```python
from build123d import *

# Parameters (mm, degrees)
SKETCH1_W               = 100
SKETCH1_H               = 240
SKETCH1_R               = 8
SKETCH1_R_2             = 10
BOSS_EXTRUDE1_DEPTH     = 25
SKETCH2_OUTSIDE_W       = 154.952
SKETCH2_OUTSIDE_H       = 294.952
SKETCH2_OUTSIDE_R       = 10
SKETCH2_OUTSIDE_R_2     = 8
CUT_EXTRUDE1_DEPTH      = 10
CUT_EXTRUDE2_START      = -50
SKETCH3_OUTSIDE_W       = 154.952
SKETCH3_OUTSIDE_H       = 294.952
CUT_EXTRUDE2_DEPTH      = 50
CUT_EXTRUDE7_REACH      = 242
SKETCH8_R               = 8
BOSS_EXTRUDE2_DEPTH     = 30
CUT_EXTRUDE8_REACH      = 242
CUT_EXTRUDE8_END_RADIUS = 115
CUT_EXTRUDE9_START      = -25.8
SKETCH10_R              = 5
CUT_EXTRUDE9_DEPTH      = 25.8
LPATTERN1_COUNT         = 4
LPATTERN1_PITCH         = 55
MIRROR1_START           = -25.8
MIRROR1_COPY_1_SKETCH_R = 5
MIRROR1_COPY_1_DEPTH    = 25.8
MIRROR1_COPY_2_SKETCH_R = 5
MIRROR1_COPY_2_DEPTH    = 25.8
MIRROR1_COPY_3_SKETCH_R = 5
MIRROR1_COPY_3_DEPTH    = 25.8
FILLET1_R               = 5


with BuildPart() as part:
    # Sketch1 → Boss-Extrude1 (new body, symmetric)
    with BuildSketch(Plane.XY):
        Rectangle(SKETCH1_W, SKETCH1_H)
        with Locations((0, 3)):
            Circle(SKETCH1_R, mode=Mode.SUBTRACT)
        with Locations((0, -85)):
            Circle(SKETCH1_R_2, mode=Mode.SUBTRACT)
    extrude(amount=BOSS_EXTRUDE1_DEPTH, both=True)

    # Sketch2 outside → Cut-Extrude1 (cut)
    with BuildSketch(Plane.XY.offset(25)):
        Rectangle(SKETCH2_OUTSIDE_W, SKETCH2_OUTSIDE_H)
        with BuildLine():
            Line((50, -120), (50, 18.561575886))
            ThreePointArc((50, 18.561575886), (0, 30), (-50, 18.561575886))
            Line((-50, 18.561575886), (-50, -120))
            Line((-50, -120), (50, -120))
        make_face(mode=Mode.SUBTRACT)
        with Locations((0, -85)):
            Circle(SKETCH2_OUTSIDE_R)
        with Locations((0, 3)):
            Circle(SKETCH2_OUTSIDE_R_2)
    extrude(amount=-CUT_EXTRUDE1_DEPTH, mode=Mode.SUBTRACT)

    # Sketch3 outside → Cut-Extrude2 (cut)
    with BuildSketch(Plane.XY.offset(25).offset(CUT_EXTRUDE2_START)):
        Rectangle(SKETCH3_OUTSIDE_W, SKETCH3_OUTSIDE_H)
        with BuildLine():
            Line((50, 120), (-50, 120))
            Line((-50, 120), (-50, -109.378823628))
            ThreePointArc((-50, -109.378823628), (0, -120), (50, -109.378823628))
            Line((50, -109.378823628), (50, 120))
        make_face(mode=Mode.SUBTRACT)
    extrude(amount=CUT_EXTRUDE2_DEPTH, mode=Mode.SUBTRACT)

    # Sketch7 → Cut-Extrude7 (cut, up to next)
    with BuildSketch(Plane(origin=(0, 120, 0), x_dir=(1, 0, 0), z_dir=(0, 1, 0)), mode=Mode.PRIVATE) as cut_extrude7_sk1:
        Polygon((-35, 0), (35, 0), (20, 25), (-20, 25), align=None)
    cut_extrude7_tool1 = extrude(cut_extrude7_sk1.sketch, amount=-CUT_EXTRUDE7_REACH, mode=Mode.PRIVATE) & part.part
    add(cut_extrude7_tool1.solids().sort_by_distance((0, 120, -11.363636))[0], mode=Mode.SUBTRACT)

    # Sketch8 → Boss-Extrude2 (add)
    with BuildSketch(Plane(origin=(0, 120, 0), x_dir=(1, 0, 0), z_dir=(0, 1, 0))):
        with BuildLine():
            Line((13, 15), (13, 0))
            Line((13, 0), (-13, 0))
            Line((-13, 0), (-13, 15))
            ThreePointArc((-13, 15), (0, 28), (13, 15))
        make_face()
        with Locations(Location((0, 15, 0), (0, 0, 270))):  # turned: the seam where the file's is
            Circle(SKETCH8_R, mode=Mode.SUBTRACT)
    extrude(amount=-BOSS_EXTRUDE2_DEPTH)

    # Cut-Extrude8: up to this cylinder (the profile starts outside it)
    cut_extrude8_end = Plane(origin=(0, -85, 18.800927), z_dir=(0, 0, 1)) * Cylinder(CUT_EXTRUDE8_END_RADIUS, 715, mode=Mode.PRIVATE)
    # Sketch9 → Cut-Extrude8 (cut, up to the surface)
    with BuildSketch(Plane(origin=(0, 120, 0), x_dir=(1, 0, 0), z_dir=(0, 1, 0)), mode=Mode.PRIVATE) as cut_extrude8_sk1:
        with BuildLine():
            Line((50, -8.64916731), (50, -25))
            Line((50, -25), (-50, -25))
            Line((-50, -25), (-50, -8.64916731))
            ThreePointArc((-50, -8.64916731), (0, -15), (50, -8.64916731))
        make_face()
    cut_extrude8_tool1 = extrude(cut_extrude8_sk1.sketch, amount=-CUT_EXTRUDE8_REACH, mode=Mode.PRIVATE) - cut_extrude8_end
    add(cut_extrude8_tool1.solids().sort_by_distance((0, 120, 18.800927))[0], mode=Mode.SUBTRACT)

    # Sketch10 → Cut-Extrude9 (cut)
    with BuildSketch(Plane(origin=(50, 0, 0), x_dir=(0, 0, -1), z_dir=(1, 0, 0)).offset(CUT_EXTRUDE9_START)):
        with Locations((13, -90)):
            Circle(SKETCH10_R)
    cut_extrude9 = extrude(amount=CUT_EXTRUDE9_DEPTH, mode=Mode.SUBTRACT)

    # LPattern1: Cut-Extrude9 ×4
    with Locations(*[(0, i * LPATTERN1_PITCH, 0) for i in range(1, LPATTERN1_COUNT)]):
        add(cut_extrude9, mode=Mode.SUBTRACT)

    # Mirror1: Cut-Extrude9 across plane
    add(cut_extrude9.mirror(Plane(origin=(0, 0, 0), x_dir=(0, 0, 1), z_dir=(1, 0, 0))), mode=Mode.SUBTRACT)

    # Mirror1 copy 1 sketch → Mirror1 copy 1 (cut)
    with BuildSketch(Plane(origin=(-50, 55, 0), x_dir=(0, 0, -1), z_dir=(-1, 0, 0)).offset(MIRROR1_START)):
        with Locations((13, 90)):
            Circle(MIRROR1_COPY_1_SKETCH_R)
    extrude(amount=MIRROR1_COPY_1_DEPTH, mode=Mode.SUBTRACT)

    # Mirror1 copy 2 sketch → Mirror1 copy 2 (cut)
    with BuildSketch(Plane(origin=(-50, 110, 0), x_dir=(0, 0, -1), z_dir=(-1, 0, 0)).offset(MIRROR1_START)):
        with Locations((13, 90)):
            Circle(MIRROR1_COPY_2_SKETCH_R)
    extrude(amount=MIRROR1_COPY_2_DEPTH, mode=Mode.SUBTRACT)

    # Mirror1 copy 3 sketch → Mirror1 copy 3 (cut)
    with BuildSketch(Plane(origin=(-50, 165, 0), x_dir=(0, 0, -1), z_dir=(-1, 0, 0)).offset(MIRROR1_START)):
        with Locations((13, 90)):
            Circle(MIRROR1_COPY_3_SKETCH_R)
    extrude(amount=MIRROR1_COPY_3_DEPTH, mode=Mode.SUBTRACT)

    # Fillet1
    fillet1_edges = [part.edges().sort_by_distance(p)[0] for p in [
        (-1e-09, 30, 15),
    ]]
    fillet(fillet1_edges, radius=FILLET1_R)


solid = part.part
```
Work out the finished part from the listing and answer in its coordinate system (mm). A direction names the side the tool comes from. Give positions to 0.01 mm unless a question says otherwise; leave off trailing zeros. Loops run counter-clockwise (first coordinate to the right, second up) from the corner with the lowest first, then second, coordinate; pieces in that order, holes last. Notation, with made-up numbers: (30, 61) -> (35, 61) arc R10 cw to (35, 66) -> close; hole circle Ø4 at (41.5, 58.25). An arc over 180 degrees is marked (long way). Put each result on its own line as item: value. Start each with the question number.
Item 1: The part is cut by section A-A (y = 75). Give the vertices of the cut face in (x, z), then the cut area to 3 significant figures.
Item 2: The mould has two halves that part along Z. Classify faces 4 (the face through (-35, 2, -25)), 5 (the face through (39.786, -36.915, -17.619)), 6 (the face through (50, 4, -5)): released by +Z, released by -Z, zero draft, split by the parting line, or undercut.
Item 3: Each of these flat-tipped pins is pushed along its axis until it touches: P1, Ø1, axis at x = 34.5, z = -17, coming from the -Y side; P2, Ø21, axis at x = 14, y = 36.5, coming from the -Z side; P3, Ø8, axis at x = 5.5, y = 70, coming from the +Z side. Where does it stop, or does it pass through?
Item 4: The part is cut by section C-C (y = 105). Give the vertices of the cut face in (x, z).
Item 5: Which of the six approach directions +Z, -Z, +X, -X, +Y, -Y give full straight-line access (tool end or side, diameter ignored) to faces 1 (the face through (6, 90, -8)), 2 (the face through (13, 105, -8)), 3 (the face through (-8.3, 1.7, 0))?
Item 6: The part is cut by section D-D (y = -102). Give the vertices of the cut face in (x, z), then the cut area to 4 significant figures.
Item 7: The part is cut by section B-B (z = 22.5). Give the vertices of the cut face in (x, y), then the cut area to 3 significant figures.
Item 8: Find the intervals of material crossed by L1, parallel to Z at x = -36.75, y = -35; L2, parallel to X at y = 91.5, z = -6.5; L3, parallel to Y at x = 0, z = 6, in increasing order. Write a range as [from, to].
Answers below:
1. outline: (-50, -25) -> (-20, -25) -> (-24.2, -18) -> (-50, -18) -> close; (-50, -8) -> (-30.2, -8) -> (-35, 0) -> (35, 0) -> (30.2, -8) -> (50, -8) -> (50, 8.65) arc R200 ccw to (-50, 8.65) -> close; (20, -25) -> (50, -25) -> (50, -18) -> (24.2, -18) -> close
1. area: 1,960 mm2
2. face 4: released by -Z
2. face 5: undercut
2. face 6: zero draft
3. P1: y = -115.21
3. P2: z = -25
3. P3: z = 14.99
4. outline: (-50, -25) -> (-20, -25) -> (-35, 0) -> (-13, 0) -> (-13, -15) arc R13 ccw to (13, -15) -> (13, 0) -> (35, 0) -> (20, -25) -> (50, -25) -> (50, 8.65) arc R200 ccw to (-50, 8.65) -> close; hole circle Ø16 at (0, -15)
5. face 1: -Z, -Y
5. face 2: -Z, +Y, -Y
5. face 3: -Y
6. outline: (-50, -25) -> (-20, -25) -> (-35, 0) -> (35, 0) -> (20, -25) -> (50, -25) -> (50, 25) -> (-50, 25) -> close
6. area: 3,625 mm2
7. outline: (-50, -109.38) arc R123 ccw to (50, -109.38) -> (50, 18.56) arc R115 ccw to (-50, 18.56) -> close; hole circle Ø20 at (0, -85); hole circle Ø16 at (0, 3)
7. area: 13,800 mm2
8. L1: [-25, -18], [-8, 25]
8. L2: [-50, -31.1], [-13, 13], [31.1, 50]
8. L3: [-120, -95], [-75, -5], [11, 120]
